from build123d import *

# Parameters (mm, degrees)
EXTRUDE_THIN1_DEPTH = 19
CUT_EXTRUDE1_DEPTH  = 60.674114991
SKETCH3_R           = 4.5
CUT_EXTRUDE2_DEPTH  = 60.674114991
BOSS_EXTRUDE1_DEPTH = 3


with BuildPart() as part:
    # Sketch1 → Extrude-Thin1 (new, symmetric)
    with BuildSketch(Plane(origin=(0, 0, 0), x_dir=(1, 0, 0), z_dir=(0, 1, 0))):
        Polygon((-40, 0), (0, 0), (0, 40), (-5, 40), (-5, 5), (-40, 5), align=None)
    extrude(amount=EXTRUDE_THIN1_DEPTH, both=True)

    # Sketch2 → Cut-Extrude1 (cut, through all)
    with BuildSketch(Plane(origin=(0, 0, 0), x_dir=(0, 0, -1), z_dir=(1, 0, 0))):
        with BuildLine():
            Line((13, 4.5), (28, 4.5))
            ThreePointArc((28, 4.5), (32.5, 0), (28, -4.5))
            Line((28, -4.5), (13, -4.5))
            ThreePointArc((13, -4.5), (8.5, 0), (13, 4.5))
        make_face()
    extrude(amount=-CUT_EXTRUDE1_DEPTH, mode=Mode.SUBTRACT)

    # Sketch3 → Cut-Extrude2 (cut, through all)
    with BuildSketch(Plane.XY):
        with Locations((-20, 0)):
            Circle(SKETCH3_R)
    extrude(amount=-CUT_EXTRUDE2_DEPTH, mode=Mode.SUBTRACT)

    # Sketch4 → Boss-Extrude1 (add)
    with BuildSketch(Plane(origin=(0, 19, 0), x_dir=(1, 0, 0), z_dir=(0, 1, 0))):
        Polygon((-38, 5), (-5, 38), (-5, 5), align=None)
    boss_extrude1 = extrude(amount=-BOSS_EXTRUDE1_DEPTH)

    # Mirror1: Boss-Extrude1 across plane
    add(boss_extrude1.mirror(Plane.ZX))


solid = part.part
Work out the finished part from the listing and answer in its coordinate system (mm). A direction names the side the tool comes from. Coordinates: 2 decimals unless noted, no trailing zeros. Write each loop counter-clockwise with the first axis right and the second up, starting at its lowest first coordinate (ties: lowest second). Pieces come first, ordered by that corner, then holes.
1. Consider line 1 along Y through (x, z) = (-20, -1.2); line 2 along Y through (x, z) = (-22.5, -8.5); line 3 along Z through (x, y) = (-24.5, 10). Determine where each line is inside the solid, lowest interval first.
Results list:
line 1: y = -19 to -4.5, 4.5 to 19
line 2: y = -19 to -16, 16 to 19
line 3: z = -5 to 0
2. For faces 1 (the flat face through (-2, -4.5, -21)), 2 (the flat face through (-22, 18, -21)), 3 (the flat face through (-5, 4, -31)), determine the directions among +Z, -Z, +X, -X, +Y, -Y from which every point of the face is accessible in a straight line to the end or side of a thin tool.
Results list:
face 1: +X, -X
face 2: -Z, -X, +Y, -Y
face 3: -Z, -X
3. The part is cut by section D-D, the plane x = -27. Write down the section's boundary in (y, z), and give its area (3 significant figures).
Results list:
outline: (-19, -16) - (-16, -16) - (-16, -5) - (16, -5) - (16, -16) - (19, -16) - (19, 0) - (-19, 0) - close
area: 256 mm2
4. The part is cut by section B-B, the plane y = 0. Write down the section's boundary in (x, z), and give its area (3 significant figures).
Results list:
outline: (-40, -5) - (-24.5, -5) - (-24.5, 0) - (-40, 0) - close; (-15.5, -5) - (-5, -5) - (-5, -8.5) - (0, -8.5) - (0, 0) - (-15.5, 0) - close; (-5, -40) - (0, -40) - (0, -32.5) - (-5, -32.5) - close
area: 210 mm2
5. Flat-ended cylindrical pins translate along their axes: pin 1 (3 mm diameter, centred on x = -24, y = 6, fed in from -Z); pin 2 (10.5 mm diameter, centred on y = 9.5, z = -21, fed in from -X). Find the tip coordinate at first contact, or state that the pin passes through.
Results list:
pin 1: stops at z = -5
pin 2: stops at x = -5
6. For a pull along Y with two mould halves and no side action, classify faces 4 (the flat face through (0, 9, -20)), 5 (the flat face through (-15, -19, -16)), 6 (the cylindrical face through (-2.5, 0.1, -32.5)) as +Y half, -Y half, draft (parallel to the pull), parting line (faces both ways), or undercut.
Results list:
face 4: draft
face 5: -Y half
face 6: undercut
7. The part is cut by section C-C, the plane x = -20. Write down the section's boundary in (y, z).
Results list:
outline: (-19, -23) - (-16, -23) - (-16, -5) - (-4.5, -5) - (-4.5, 0) - (-19, 0) - close; (4.5, -5) - (16, -5) - (16, -23) - (19, -23) - (19, 0) - (4.5, 0) - close
8. The part is cut by section A-A, the plane z = -14. Write down the section's boundary in (x, y), and give its area (3 significant figures).
Results list:
outline: (-29, -19) - (0, -19) - (0, -4.5) - (-5, -4.5) - (-5, -16) - (-29, -16) - close; (-29, 16) - (-5, 16) - (-5, 4.5) - (0, 4.5) - (0, 19) - (-29, 19) - close
area: 289 mm2
